Job drawing, mm, ordinate dimensions from the low corner. One solid piece. A direction names the side the tool comes from. Give positions to 0.01 mm unless a question says otherwise; leave off trailing zeros. Order: outer loops, then holes, each group sorted by start corner. A loop starts at its lowest first (then second) coordinate and runs counter-clockwise, first axis right, second up. Notation, with made-up numbers: M 84,86.5 L 107,86.5 A29 ccw 107,107.5 Z; hole C 53.25,2 d11. An arc over 180 degrees is marked long. Put each result on its own line as item: value. Start each with the question number.
1) Drill centre lines: line 1 (X direction, y = 3.75, z = 38.6); line 2 (Z direction, x = 6.7, y = 4.3); line 3 (Z direction, x = 69.25, y = 1.9). Where is each one in solid material? Low to high. Write a range as [from, to].
2) Cut at A-A (z = 38.6). Write the cut outline in (x, y).
3) Cut at D-D (x = 69.25). Write the cut outline in (y, z).
4) Cut at B-B (x = 6.7). Write the cut outline in (y, z), and give its area (3 significant figures).
5) Tool access for the marked faces 1, 2 and 3: list every direction of +Z, -Z, +X, -X, +Y, -Y with a clear straight run to the whole face (end or side of a thin tool).
6) Pin check, flat tips, straight feed: pin 1 (2 mm diameter, centred on y = 1, z = 52, fed in from -X) (1 decimal); pin 2 (1.8 mm diameter, centred on x = 14.5, y = 4, fed in from -Z); pin 3 (1.5 mm diameter, centred on x = 20, z = 48, fed in from -Y); pin 4 (3 mm diameter, centred on y = 3.5, z = 32, fed in from -X). Stop position of each tip, or through.
7) Two-plate mould, pull along X, no slides. Class the marked faces 4, 5 and 6: released by +X, released by -X, zero draft, split by the parting line, or undercut.
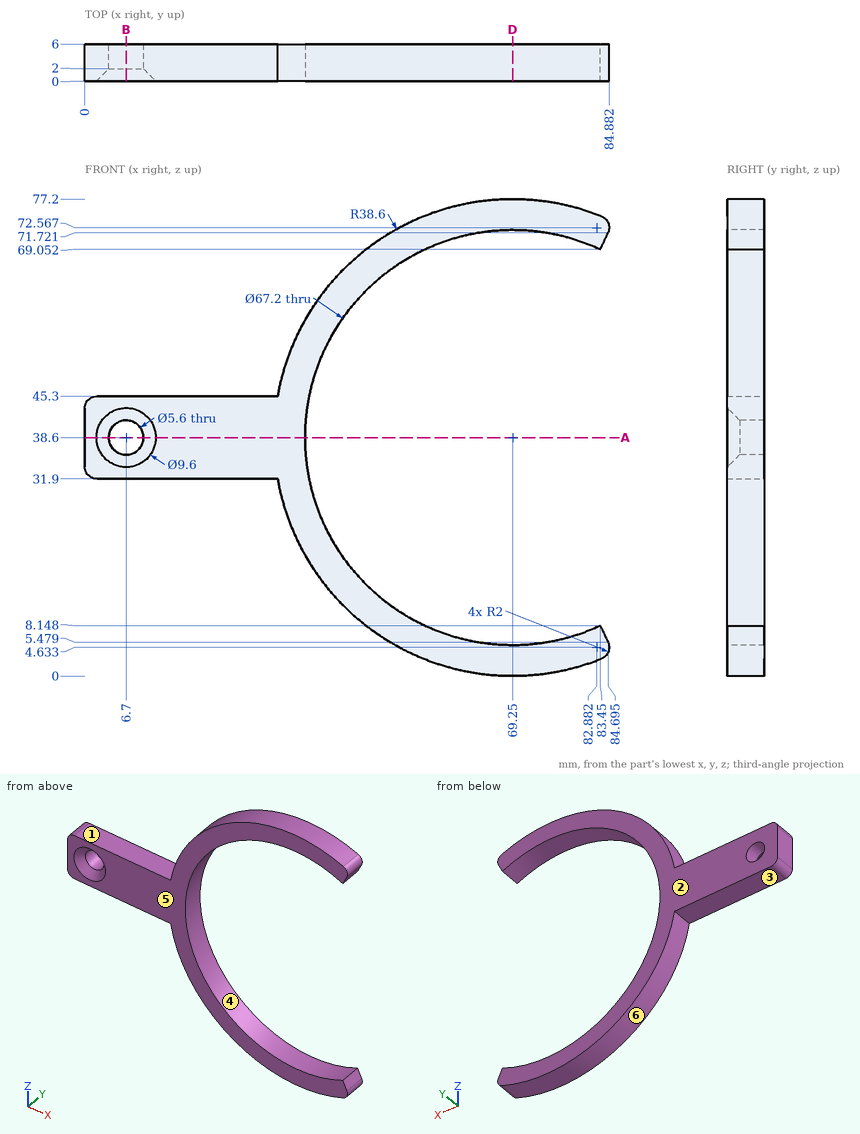
Solution:
1. line 1: [0, 3.9], [9.5, 35.65]
1. line 2: [31.9, 35.8], [41.4, 45.3]
1. line 3: [0, 5], [72.2, 77.2]
2. outline: M 0,0 L 1.9,0 L 3.9,2 L 3.9,6 L 0,6 Z; M 9.5,2 L 11.5,0 L 35.65,0 L 35.65,6 L 9.5,6 Z
3. outline: M 0,0 L 6,0 L 6,5 L 0,5 Z; M 0,72.2 L 6,72.2 L 6,77.2 L 0,77.2 Z
4. outline: M 0,31.9 L 6,31.9 L 6,35.8 L 2,35.8 L 0,33.8 Z; M 0,43.4 L 2,41.4 L 6,41.4 L 6,45.3 L 0,45.3 Z
4. area: 42.8 mm²
5. face 1: +Z, -X, +Y, -Y
5. face 2: +Z, -Z, +X, -X, +Y
5. face 3: -Z, -X, +Y, -Y
6. pin 1: x = 32.7
6. pin 2: z = 31.9
6. pin 3: through
6. pin 4: x = 0.04
7. face 4: undercut
7. face 5: zero draft
7. face 6: split by the parting line
